Design review of the part built by this model. Coordinates are the model's own, in mm. A direction names the side the tool comes from. Round coordinates to 2 decimals unless told otherwise and drop trailing zeros. Order: outer loops, then holes, each group sorted by start corner. A loop starts at its lowest first (then second) coordinate and runs counter-clockwise, first axis right, second up. Notation, with made-up numbers: (4.5, -35) - (39.5, -35) arc R7 cw to (39.5, -30) - close; hole circle Ø7 at (82, 8.25). An arc over 180 degrees is marked (long way). Write item = value, one per line.
from build123d import *

# Parameters (mm, degrees)
BASPROSKE_W        = 13
BASPROSKE_H        = 10.5
TOOTHCUT_DEPTH     = 20.735754356
TEETHCUTS_COUNT    = 10
TEETHCUTS_ANGLE    = 324
BORSKE_R           = 1.5
BORE_DEPTH         = 50.0000508
SKETCH1_R          = 4.05
CUT_EXTRUDE1_DEPTH = 3
CUT_EXTRUDE2_REACH = 19.646
SKETCH2_R          = 2.25
CHAMFER1_SIZE      = 0.5


with BuildPart() as part:
    # BasProSke → Base-Revolve (revolve)
    with BuildSketch(Plane(origin=(0, 0, 0), x_dir=(1, 0, 0), z_dir=(0, 1, 0)), mode=Mode.PRIVATE) as base_revolve_sk:
        with Locations((6.5, 5.25)):
            Rectangle(BASPROSKE_W, BASPROSKE_H)
    revolve(base_revolve_sk.sketch.rotate(Axis((-10, 0, 0), (1, 0, 0)), 180), axis=Axis((-10, 0, 0), (1, 0, 0)))

    # TooCutSke → ToothCut (cut, through all)
    with BuildSketch(Plane(origin=(0, 0, 0), x_dir=(0, 0, -1), z_dir=(1, 0, 0))):
        with BuildLine():
            ThreePointArc((1.019600066, 6.481797432), (0, 6.5615), (-1.019600066, 6.481797432))
            ThreePointArc((-1.019600066, 6.481797432), (-1.451036104, 8.608938557), (-3.053606956, 10.072712133))
            ThreePointArc((-3.053606956, 10.072712133), (0, 10.5254), (3.053606956, 10.072712133))
            ThreePointArc((3.053606956, 10.072712133), (1.451036104, 8.608938557), (1.019600066, 6.481797432))
        make_face()
    toothcut = extrude(amount=TOOTHCUT_DEPTH, mode=Mode.SUBTRACT)

    # TeethCuts: ToothCut ×10 about axis
    teethcuts_axis = Axis((-10, 0, 0), (1, 0, 0))
    for i in range(1, TEETHCUTS_COUNT):
        add(toothcut.rotate(teethcuts_axis, i * TEETHCUTS_ANGLE / (TEETHCUTS_COUNT - 1)), mode=Mode.SUBTRACT)

    # BorSke → Bore (cut, symmetric)
    with BuildSketch(Plane(origin=(0, 0, 0), x_dir=(0, 0, -1), z_dir=(1, 0, 0))):
        with Locations(Location((0, 0, 0), (0, 0, 180))):
            Circle(BORSKE_R)
    extrude(amount=BORE_DEPTH, both=True, mode=Mode.SUBTRACT)

    # Sketch1 → Cut-Extrude1 (cut)
    with BuildSketch(Plane.ZY):
        Circle(SKETCH1_R)
    cut_extrude1 = extrude(amount=-CUT_EXTRUDE1_DEPTH, mode=Mode.SUBTRACT)

    # Mirror1: Cut-Extrude1 across plane
    add(cut_extrude1.mirror(Plane(origin=(6.5, 0, 0), x_dir=(0, 0, 1), z_dir=(1, 0, 0))), mode=Mode.SUBTRACT)

    # Sketch2 → Cut-Extrude2 (cut, up to next)
    with BuildSketch(Plane(origin=(10, 0, 0), x_dir=(0, 0, -1), z_dir=(1, 0, 0)), mode=Mode.PRIVATE) as cut_extrude2_sk1:
        Circle(SKETCH2_R)
    cut_extrude2_tool1 = extrude(cut_extrude2_sk1.sketch, amount=-CUT_EXTRUDE2_REACH, mode=Mode.PRIVATE) & part.part
    add(cut_extrude2_tool1.solids().sort_by_distance((10, 0, 0))[0], mode=Mode.SUBTRACT)

    # Chamfer1
    chamfer1_edges = [part.edges().sort_by_distance(p)[0] for p in [
        (0, 0, -4.05),
        (13, 0, -4.05),
        (3, 0, 2.25),
        (10, 0, 2.25),
    ]]
    chamfer(chamfer1_edges, length=CHAMFER1_SIZE)


solid = part.part
1) We need section A-A on z = 0. Write out the cut boundary in (x, y), and give its area (3 significant figures).
Findings:
outline = (0, -6.56) - (13, -6.56) - (13, -4.55) - (12.5, -4.05) - (10, -4.05) - (10, -2.75) - (9.5, -2.25) - (3.5, -2.25) - (3, -2.75) - (3, -4.05) - (0.5, -4.05) - (0, -4.55) - close; (0, 4.55) - (0.5, 4.05) - (3, 4.05) - (3, 2.75) - (3.5, 2.25) - (9.5, 2.25) - (10, 2.75) - (10, 4.05) - (12.5, 4.05) - (13, 4.55) - (13, 6.56) - (0, 6.56) - close
area = 89.5 mm^2
2) For faces 1 (the cylindrical face through (11.268, -3.954, -0.878)), 2 (the cylindrical face through (6.54, 2.23, 0.29)), list the 3-axis set-ups (+Z, -Z, +X, -X, +Y, -Y) from which the entire face can be reached by the end or side of a thin tool; tool diameter is ignored.
Findings:
face_1 = +X
face_2 = +X, -X
3) The part is to be moulded in two halves that separate along Z. For faces 3 (the cylindrical face through (6.409, 1.278, -8.647)), 4 (the flat face through (13, -5, 0)), say which applies: released by +Z, released by -Z, zero draft, split by the parting line, or undercut.
Findings:
face_3 = undercut
face_4 = zero draft
4) Clearance check with flat-ended pins moving along their axes: pin 1 Ø6 at (x, z) = (9, 8) entering from -Y; pin 2 Ø4 at (y, z) = (2, 1.5) entering from -X; pin 3 Ø3 at (x, z) = (7.5, 1) entering from +Y. State where each tip first meets the part, or that it passes through.
Findings:
pin_1 = -6.43
pin_2 = 0.05
pin_3 = 9.76
5) We need section B-B on y = 7.5. Write out the cut boundary in (x, z).
Findings:
outline = (0, -3.84) - (13, -3.84) - (13, -1.05) - (0, -1.05) - close; (0, 1.05) - (13, 1.05) - (13, 3.84) - (0, 3.84) - close
6) To check wall thickness, follow L1, parallel to Y at x = 6.95, z = 0; L2, parallel to Y at x = 1.5, z = 0; L3, parallel to Y at x = 8, z = 3.25. State the ranges of each line that lie inside material, in increasing order. Write a range as from..to.
Findings:
L1 = -6.56..-2.25, 2.25..6.56
L2 = -6.56..-4.05, 4.05..6.56
L3 = -9.98..-6.17, -5.7..5.7, 6.17..9.98
7) We need section C-C on y = -5. Write out the cut boundary in (x, z), and give its area (3 significant figures).
Findings:
outline = (0, -8.36) - (13, -8.36) - (13, -4.86) - (0, -4.86) - close; (0, -4.25) - (13, -4.25) - (13, 4.25) - (0, 4.25) - close; (0, 4.86) - (13, 4.86) - (13, 8.36) - (0, 8.36) - close
area = 201 mm^2
